Part model, mm, in its own coordinate system. A direction names the side the tool comes from. Coordinates: 2 decimals unless noted, no trailing zeros. Write each question's results on one line, items separated by ' | '.
from build123d import *

# Parameters (mm, degrees)
BOSS_EXTRU_1_DEPTH      = 10
BOSS_EXTRU_1_DEPTH_BACK = 10
ESQUISSE1_W             = 20
ESQUISSE1_H             = 110
ESQUISSE2_R             = 2.1
ENL_V_MAT_EXTRU_1_DEPTH = 111.905365064


with BuildPart() as part:
    # Esquisse1 → Boss.-Extru.1 (new, two sides: drawn at the far end of the back side and taken through both)
    with BuildSketch(Plane.XY.offset(-BOSS_EXTRU_1_DEPTH_BACK)):
        Rectangle(ESQUISSE1_W, ESQUISSE1_H)
    extrude(amount=BOSS_EXTRU_1_DEPTH + BOSS_EXTRU_1_DEPTH_BACK)

    # Esquisse2 → Enl_v. mat.-Extru.1 (cut, through all)
    with BuildSketch(Plane(origin=(0, 55, 0), x_dir=(1, 0, 0), z_dir=(0, 1, 0))):
        with BuildLine():
            Line((-3.441421356, -8.641421356), (-4.8, -10))
            Line((-4.8, -10), (4.8, -10))
            Line((4.8, -10), (3.441421356, -8.641421356))
            ThreePointArc((3.441421356, -8.641421356), (3.398066806, -8.423463314), (3.582842712, -8.3))
            Line((3.582842712, -8.3), (5.3, -8.3))
            ThreePointArc((5.3, -8.3), (5.441421356, -8.241421356), (5.5, -8.1))
            Line((5.5, -8.1), (5.5, -6.560660172))
            Line((5.5, -6.560660172), (2.939339828, -4))
            Line((2.939339828, -4), (0.282842712, -4))
            Line((0.282842712, -4), (0, -3.717157288))
            Line((0, -3.717157288), (-0.282842712, -4))
            Line((-0.282842712, -4), (-2.939339828, -4))
            Line((-2.939339828, -4), (-5.5, -6.560660172))
            Line((-5.5, -6.560660172), (-5.5, -8.1))
            ThreePointArc((-5.5, -8.1), (-5.441421356, -8.241421356), (-5.3, -8.3))
            Line((-5.3, -8.3), (-3.582842712, -8.3))
            ThreePointArc((-3.582842712, -8.3), (-3.398066806, -8.423463314), (-3.441421356, -8.641421356))
        make_face()
        with BuildLine():
            Line((-10, 4.8), (-10, -4.8))
            Line((-10, -4.8), (-8.641421356, -3.441421356))
            ThreePointArc((-8.641421356, -3.441421356), (-8.423463314, -3.398066806), (-8.3, -3.582842712))
            Line((-8.3, -3.582842712), (-8.3, -5.3))
            ThreePointArc((-8.3, -5.3), (-8.241421356, -5.441421356), (-8.1, -5.5))
            Line((-8.1, -5.5), (-6.560660172, -5.5))
            Line((-6.560660172, -5.5), (-4, -2.939339828))
            Line((-4, -2.939339828), (-4, -0.282842712))
            Line((-4, -0.282842712), (-3.717157288, 0))
            Line((-3.717157288, 0), (-4, 0.282842712))
            Line((-4, 0.282842712), (-4, 2.939339828))
            Line((-4, 2.939339828), (-6.560660172, 5.5))
            Line((-6.560660172, 5.5), (-8.1, 5.5))
            ThreePointArc((-8.1, 5.5), (-8.241421356, 5.441421356), (-8.3, 5.3))
            Line((-8.3, 5.3), (-8.3, 3.582842712))
            ThreePointArc((-8.3, 3.582842712), (-8.423463314, 3.398066806), (-8.641421356, 3.441421356))
            Line((-8.641421356, 3.441421356), (-10, 4.8))
        make_face()
        with BuildLine():
            Line((8.641421356, -3.441421356), (10, -4.8))
            Line((10, -4.8), (10, 4.8))
            Line((10, 4.8), (8.641421356, 3.441421356))
            ThreePointArc((8.641421356, 3.441421356), (8.423463314, 3.398066806), (8.3, 3.582842712))
            Line((8.3, 3.582842712), (8.3, 5.3))
            ThreePointArc((8.3, 5.3), (8.241421356, 5.441421356), (8.1, 5.5))
            Line((8.1, 5.5), (6.560660172, 5.5))
            Line((6.560660172, 5.5), (4, 2.939339828))
            Line((4, 2.939339828), (4, 0.282842712))
            Line((4, 0.282842712), (3.717157288, 0))
            Line((3.717157288, 0), (4, -0.282842712))
            Line((4, -0.282842712), (4, -2.939339828))
            Line((4, -2.939339828), (6.560660172, -5.5))
            Line((6.560660172, -5.5), (8.1, -5.5))
            ThreePointArc((8.1, -5.5), (8.241421356, -5.441421356), (8.3, -5.3))
            Line((8.3, -5.3), (8.3, -3.582842712))
            ThreePointArc((8.3, -3.582842712), (8.423463314, -3.398066806), (8.641421356, -3.441421356))
        make_face()
        with BuildLine():
            Line((4.8, 10), (-4.8, 10))
            Line((-4.8, 10), (-3.441421356, 8.641421356))
            ThreePointArc((-3.441421356, 8.641421356), (-3.398066806, 8.423463314), (-3.582842712, 8.3))
            Line((-3.582842712, 8.3), (-5.3, 8.3))
            ThreePointArc((-5.3, 8.3), (-5.441421356, 8.241421356), (-5.5, 8.1))
            Line((-5.5, 8.1), (-5.5, 6.560660172))
            Line((-5.5, 6.560660172), (-2.939339828, 4))
            Line((-2.939339828, 4), (-0.282842712, 4))
            Line((-0.282842712, 4), (0, 3.717157288))
            Line((0, 3.717157288), (0.282842712, 4))
            Line((0.282842712, 4), (2.939339828, 4))
            Line((2.939339828, 4), (5.5, 6.560660172))
            Line((5.5, 6.560660172), (5.5, 8.1))
            ThreePointArc((5.5, 8.1), (5.441421356, 8.241421356), (5.3, 8.3))
            Line((5.3, 8.3), (3.582842712, 8.3))
            ThreePointArc((3.582842712, 8.3), (3.398066806, 8.423463314), (3.441421356, 8.641421356))
            Line((3.441421356, 8.641421356), (4.8, 10))
        make_face()
        with Locations(Location((0, 0, 0), (0, 0, 270))):
            Circle(ESQUISSE2_R)
    extrude(amount=-ENL_V_MAT_EXTRU_1_DEPTH, mode=Mode.SUBTRACT)


solid = part.part
(1) Wall check: line 1 (Z direction, x = -4.5, y = 30); line 2 (Z direction, x = 4.25, y = 36); line 3 (X direction, y = -32, z = 8.5). Give the ranges that are in metal, low to high. Write a range as from..to.
Return value:
line 1: z = -9.7..-8.3, -5.56..-3.44, 3.44..5.56, 8.3..9.7 | line 2: z = -9.45..-8.3, -5.31..-3.19, 3.19..5.31, 8.3..9.45 | line 3: x = -10..-3.38, 3.38..10
(2) Two-plate mould, pull along X, no slides. Class faces 1 (the flat face through (4, 1, 2)), 2 (the flat face through (-4.24, 0.77, -5.3)), 3 (the flat face through (-7, 1, 10)): released by +X, released by -X, zero draft, split by the parting line, or undercut.
Return value:
face 1: released by +X | face 2: undercut | face 3: zero draft
(3) Flat gauge pins, fed straight in: P1, Ø3, axis at y = -11.5, z = -1, coming from the -X side; P2, Ø1.5, axis at x = -3.5, y = -32, coming from the -Z side; P3, Ø1.4, axis at y = 7, z = -4, coming from the -X side. Where does each tip first touch, or does it go through?
Return value:
P1: stops at x = -4 | P2: stops at z = -9.45 | P3: stops at x = -9.9
(4) 3-axis set-ups, long thin cutter, end or side, ignore diameter. For faces 4 (the flat face through (5.3, 0.77, -4.24)), 5 (the flat face through (7, 1, 10)), 6 (the flat face through (4, 1, -2)), 7 (the flat face through (-2, 1, 4)): which of +Z, -Z, +X, -X, +Y, -Y reach the whole face in a straight line?
Return value:
face 4: +Y, -Y | face 5: +Z, +X, -X, +Y, -Y | face 6: +X, +Y, -Y | face 7: +Z, +Y, -Y
